```python
from build123d import *

# Parameters (mm, degrees)
SKETCH1_R           = 12.7
SKETCH1_R_2         = 4.7625
BOSS_EXTRUDE1_DEPTH = 12.7


with BuildPart() as part:
    # Sketch1 → Boss-Extrude1 (new body)
    with BuildSketch(Plane.XY):
        with BuildLine():
            Line((-187.814837627, 239.286832502), (-109.585986317, 260.040435914))
            ThreePointArc((-109.585986317, 260.040435914), (-108.059532137, 259.226405199), (-108.761135557, 257.645120591))
            ThreePointArc((-108.761135557, 257.645120591), (-229.615919323, 149.828924192), (-260.74357991, -9.109050224))
            ThreePointArc((-260.74357991, -9.109050224), (-257.535715145, -17.439529004), (-250.885068445, -23.394037509))
            ThreePointArc((-250.885068445, -23.394037509), (-251.565109459, -68.479908862), (-288.037537466, -41.966511367))
            ThreePointArc((-288.037537466, -41.966511367), (-287.832141181, -38.557969421), (-288.238569154, -35.167517809))
            ThreePointArc((-288.238569154, -35.167517809), (-292.752508854, -7.04544043), (-294.442288596, 21.386434854))
            ThreePointArc((-294.442288596, 21.386434854), (-302.842926447, 35.611738456), (-319.362594724, 35.436984704))
            ThreePointArc((-319.362594724, 35.436984704), (-320.58266827, 34.722082272), (-321.809158258, 34.018244753))
            ThreePointArc((-321.809158258, 34.018244753), (-328.648477907, 27.400808215), (-331.433346202, 18.300738536))
            ThreePointArc((-331.433346202, 18.300738536), (-372.60107774, -0.462072999), (-363.664476838, 43.888376615))
            ThreePointArc((-363.664476838, 43.888376615), (-310.417085479, 73.549005343), (-276.36661221, 124.101976107))
            ThreePointArc((-276.36661221, 124.101976107), (-249.008169348, 178.646013909), (-210.684679592, 226.131238859))
            ThreePointArc((-210.684679592, 226.131238859), (-200.118731843, 234.219669183), (-187.814837627, 239.286832502))
        make_face()
        with Locations((-262.922494985, -45.760538404)):
            Circle(SKETCH1_R, mode=Mode.SUBTRACT)
        with Locations((-356.808175222, 19.431248244)):
            Circle(SKETCH1_R_2, mode=Mode.SUBTRACT)
    extrude(amount=BOSS_EXTRUDE1_DEPTH)


solid = part.part
```
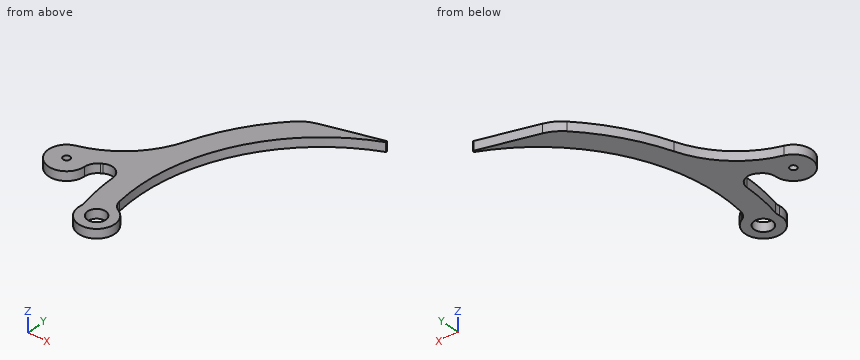
Check sheet for the modelled part. Datum: model origin and axes. Units: mm. Round coordinates to 2 decimals unless told otherwise and drop trailing zeros. Loops run counter-clockwise (first coordinate to the right, second up) from the corner with the lowest first, then second, coordinate; pieces in that order, holes last. Notation, with made-up numbers: (55, -25) - (71, -25) arc R19 cw to (71, -9) - close; hole circle Ø11 at (45.5, 83). An arc over 180 degrees is marked (long way). Write item = value, one per line. Start each with the question number.
Q1. Thickness scan on L1, parallel to Y at x = -270, z = 9.5; L2, parallel to X at y = 18, z = 5.25; L3, parallel to Y at x = -273, z = 2.25. Record the ranges inside material, lowest first.
Q2. Depth check by flat-ended pin: P1, Ø3, axis at x = -204, z = 7.5, coming from the +Y side; P2, Ø5, axis at x = -195.5, z = 3.5, coming from the +Y side. Enter the tip coordinate at first touch or a pass-through.
Q3. Section check C-C (x = -202.5). Record the boundary of the cut face in (y, z).
Q4. Section check D-D (y = 168). Record the boundary of the cut face in (x, z), plus the area to 3 significant figures.
Q5. Section check A-A (y = -49.5). Record the boundary of the cut face in (x, z).
Q6. Section check B-B (z = 10.5). Count the separate pieces of the cut face and the enclosed holes in it, plus the area to 3 significant figures.
Derived:
q1.L1 = -70.15 to -56.31, -35.22 to 139.71
q1.L2 = -382.17 to -361.35, -352.27 to -331.45, -294.39 to -262.85
q1.L3 = -69.08 to -53.49, -38.03 to 132.68
q2.P1 = 232.76
q2.P2 = 237.61
q3.outline = (188.54, 0) - (232.76, 0) - (232.76, 12.7) - (188.54, 12.7) - close
q4.outline = (-255.54, 0) - (-218.22, 0) - (-218.22, 12.7) - (-255.54, 12.7) - close
q4.area = 474 mm^2
q5.outline = (-288.05, 0) - (-275.06, 0) - (-275.06, 12.7) - (-288.05, 12.7) - close; (-250.79, 0) - (-237.8, 0) - (-237.8, 12.7) - (-250.79, 12.7) - close
q6.separate_pieces = 1
q6.enclosed_holes = 2
q6.area = 15,400 mm^2
